Geometry: final body of the model. Coordinates: model frame, mm. A direction names the side the tool comes from. Coordinates: 2 decimals unless noted, no trailing zeros. Order: outer loops, then holes, each group sorted by start corner. A loop starts at its lowest first (then second) coordinate and runs counter-clockwise, first axis right, second up. Notation, with made-up numbers: (59, -31.75) -> (93, -31.75) arc R18 ccw to (93, 0.25) -> close; hole circle Ø2 at (26, 71.25). An arc over 180 degrees is marked (long way). Answer in a Markdown table with one row per item. Add a question column.
1) Pull-direction query (Y, two-part tool) for faces 4 (the face through (747, -8, 0)), 5 (the face through (807.5, -46.8, 22.225)), 6 (the face through (747, -59.66, 19)); classes: +Y half, -Y half, draft (parallel to the pull), parting line (faces both ways), or undercut.
2) Section query C-C on z = 11.5. Count the separate pieces of the cut face and the enclosed holes in it, then the cut area to 3 significant figures.
3) Set-up query: faces 1 (the face through (691, -13, 22.225)), 2 (the face through (825, 34, 15.875)), 3 (the face through (689.994, -6.953, 10.957)). Return all of +Z, -Z, +X, -X, +Y, -Y with unobstructed straight access to the full face (end or side cutting, diameter ignored); none if empty.
4) Contact query for a flat-ended pin moving along its axis: P1, Ø6, axis at x = 832, y = 26, coming from the -Z side (3 decimals). Output: stop coordinate, or through.
5) Section query A-A on x = 805. Return the cut outline in (y, z) (3 decimals).
6) Ray query, line 1 (X direction, y = -46, z = 4); line 2 (X direction, y = 23.5, z = 34); line 3 (X direction, y = -1, z = 29.5). Return the intervals inside material, ascending. Write a range as from..to.
7) Section query B-B on y = -4.5. Return the cut outline in (x, z) (3 decimals), then the cut area to 3 significant figures.
```python
from build123d import *

# Parameters (mm, degrees)
F0_W           = 193.04
F0_H           = 101.6
F0_R           = 6.731
F0_R_2         = 10.16
F0_R_3         = 6.5278
F0_R_4         = 6.35
F1_DEPTH       = 38.1
F2_D           = 12.7
F2_DEPTH       = 50.8
F2_CBORE_D     = 20.32
F2_CBORE_DEPTH = 15.875
F2_TIP         = 3.8154649308
F4_D           = 13.462
F4_DEPTH       = 50.8
F4_TIP         = 4.0443928267
F5_D           = 12.7
F5_DEPTH       = 50.8
F5_CBORE_D     = 20.32
F5_CBORE_DEPTH = 15.875
F5_TIP         = 3.8154649308


with BuildPart() as f1:
    # F0 (on Top) → F1 (new body)
    with BuildSketch(Plane.XY):
        with Locations((748.7553224, -8.8601296)):
            Rectangle(F0_W, F0_H)
        with Locations((685.9330706, -42.1976296)):
            Circle(F0_R, mode=Mode.SUBTRACT)
        with Locations((696.0503224, -8.8601296)):
            Circle(F0_R_2, mode=Mode.SUBTRACT)
        with Locations((685.9330706, 24.4773704)):
            Circle(F0_R, mode=Mode.SUBTRACT)
        with Locations((800.8253224, -46.9601296)):
            Circle(F0_R_2, mode=Mode.SUBTRACT)
        with Locations((830.0353224, -46.9601296)):
            Circle(F0_R_2, mode=Mode.SUBTRACT)
        with Locations((765.9003224, -8.8601296)):
            Circle(F0_R_2, mode=Mode.SUBTRACT)
        with Locations((800.8253224, 29.2398704)):
            Circle(F0_R_2, mode=Mode.SUBTRACT)
        with Locations((830.0353224, 29.2398704)):
            Circle(F0_R_2, mode=Mode.SUBTRACT)
        with Locations((830.0353224, -46.9601296)):
            Circle(F0_R_2)
        with Locations((830.0353224, -46.9601296)):
            Circle(F0_R_3, mode=Mode.SUBTRACT)
        with Locations((800.8253224, 29.2398704)):
            Circle(F0_R_2)
        with Locations((800.8253224, 29.2398704)):
            Circle(F0_R_4, mode=Mode.SUBTRACT)
        with Locations((830.0353224, 29.2398704)):
            Circle(F0_R_2)
        with Locations((830.0353224, 29.2398704)):
            Circle(F0_R_3, mode=Mode.SUBTRACT)
        with Locations((696.0503224, -8.8601296)):
            Circle(F0_R_2)
        with Locations((696.0503224, -8.8601296)):
            Circle(F0_R_4, mode=Mode.SUBTRACT)
        with Locations((800.8253224, -46.9601296)):
            Circle(F0_R_2)
        with Locations((800.8253224, -46.9601296)):
            Circle(F0_R_4, mode=Mode.SUBTRACT)
        with Locations((765.9003224, -8.8601296)):
            Circle(F0_R_2)
        with Locations((765.9003224, -8.8601296)):
            Circle(F0_R_4, mode=Mode.SUBTRACT)
        with Locations((685.9330706, 24.4773704)):
            Circle(F0_R)
        with Locations((685.9330706, -42.1976296)):
            Circle(F0_R)
        with Locations((830.0353224, -46.9601296)):
            Circle(F0_R_3)
        with Locations((830.0353224, 29.2398704)):
            Circle(F0_R_3)
        with Locations((800.8253224, 29.2398704)):
            Circle(F0_R_4)
        with Locations((765.9003224, -8.8601296)):
            Circle(F0_R_4)
        with Locations((696.0503224, -8.8601296)):
            Circle(F0_R_4)
        with Locations((800.8253224, -46.9601296)):
            Circle(F0_R_4)
    extrude(amount=-F1_DEPTH)

    # F2
    with Locations(Plane.XY):
        with Locations((800.8253224, 29.2398704), (800.8253224, -46.9601296), (765.9003224, -8.8601296), (696.0503224, -8.8601296)):
            CounterBoreHole(F2_D / 2, F2_CBORE_D / 2, F2_CBORE_DEPTH, depth=F2_DEPTH)
            with Locations((0, 0, -(F2_DEPTH + F2_TIP / 2))):  # 118° drill point
                Cone(0, F2_D / 2, F2_TIP, mode=Mode.SUBTRACT)


with BuildPart() as f1_1:
    # F3: moved
    add(f1.part.moved(Location((0, 0, 38.1))))

    # F4
    with Locations(Plane(origin=(0, 0, 0), x_dir=(1, 0, 0), z_dir=(0, 0, -1))):
        with Locations((685.9330706, -24.4773704), (685.9330706, 42.1976296)):
            Hole(F4_D / 2, depth=F4_DEPTH)
            with Locations((0, 0, -(F4_DEPTH + F4_TIP / 2))):  # 118° drill point
                Cone(0, F4_D / 2, F4_TIP, mode=Mode.SUBTRACT)

    # F5
    with Locations(Plane(origin=(0, 0, 0), x_dir=(1, 0, 0), z_dir=(0, 0, -1))):
        with Locations((830.0353224, 46.9601296), (830.0353224, -29.2398704)):
            CounterBoreHole(F5_D / 2, F5_CBORE_D / 2, F5_CBORE_DEPTH, depth=F5_DEPTH)
            with Locations((0, 0, -(F5_DEPTH + F5_TIP / 2))):  # 118° drill point
                Cone(0, F5_D / 2, F5_TIP, mode=Mode.SUBTRACT)


solid = f1_1.part
```
Result:
| question | item | result |
|---|---|---|
| 1 | face 4 | draft |
| 1 | face 5 | undercut |
| 1 | face 6 | -Y half |
| 2 | separate pieces | 1 |
| 2 | enclosed holes | 8 |
| 2 | area | 18,200 mm2 |
| 3 | face 1 | +Z |
| 3 | face 2 | -Z |
| 3 | face 3 | +Z, -Z |
| 4 | P1 | z = 15.875 |
| 5 | outline | (-59.66, 0) -> (-51.745, 0) -> (-51.745, 22.225) -> (-56.223, 22.225) -> (-56.223, 38.1) -> (-59.66, 38.1) -> close; (-42.175, 0) -> (24.455, 0) -> (24.455, 22.225) -> (19.977, 22.225) -> (19.977, 38.1) -> (-37.697, 38.1) -> (-37.697, 22.225) -> (-42.175, 22.225) -> close; (34.025, 0) -> (41.94, 0) -> (41.94, 38.1) -> (38.503, 38.1) -> (38.503, 22.225) -> (34.025, 22.225) -> close |
| 6 | line 1 | 652.24..680.38, 691.49..794.55, 807.1..819.92, 840.15..845.28 |
| 6 | line 2 | 652.24..679.27, 692.59..792.44, 809.21..827.32, 832.75..845.28 |
| 6 | line 3 | 652.24..689.61, 702.49..759.46, 772.34..845.28 |
| 7 | outline | (652.235, 0) -> (691.434, 0) -> (691.434, 22.225) -> (686.873, 22.225) -> (686.873, 38.1) -> (652.235, 38.1) -> close; (700.667, 0) -> (761.284, 0) -> (761.284, 22.225) -> (756.723, 22.225) -> (756.723, 38.1) -> (705.227, 38.1) -> (705.227, 22.225) -> (700.667, 22.225) -> close; (770.517, 0) -> (845.275, 0) -> (845.275, 38.1) -> (775.077, 38.1) -> (775.077, 22.225) -> (770.517, 22.225) -> close |
| 7 | area | 6,360 mm2 |
